Job drawing, mm, ordinate dimensions from the low corner. One solid piece. A direction names the side the tool comes from. Coordinates: 2 decimals unless noted, no trailing zeros. Order: outer loops, then holes, each group sorted by start corner. A loop starts at its lowest first (then second) coordinate and runs counter-clockwise, first axis right, second up. Notation, with made-up numbers: (47, 0.5) -> (78, 0.5) arc R21 cw to (78, 8.5) -> close; hole circle Ø10 at (58, 61). An arc over 180 degrees is marked (long way). Use CSV: the item, a comma, the result in double quotes. Start each with the question number.
(1) Cut at B-B on y = 2.85. Write the cut outline in (x, z) (1 decimal).
(2) Probe L1, parallel to Z at x = 4.2, y = 4.2; L2, parallel to Z at x = 2.9, y = 5.7; L3, parallel to Y at x = 2.35, z = 10.25 (1 decimal). List the from-to ranges inside material, lowest first.
(3) Pull direction Y, two halves, no side cores. Call the marked faces 1, 2 and 3: pulls with the +Y half, pulls with the -Y half, needs draft (parallel to the pull), parting line crosses it, or undercut.
(4) Cut at C-C on z = 1.5. Write the cut outline in (x, y).
(5) Pin check, flat tips, straight feed: pin 1 Ø1.8 at (x, y) = (2.5, 3.5) entering from +Z; pin 2 Ø3 at (x, z) = (5, 8.5) entering from +Y. Stop position of each tip, or through.
(6) Cut at D-D on x = 0.6. Write the cut outline in (y, z), plus the area to 3 significant figures.
(7) Tool access for the marked faces 4, 5 and 6: list every direction of +Z, -Z, +X, -X, +Y, -Y with a clear straight run to the whole face (end or side of a thin tool).
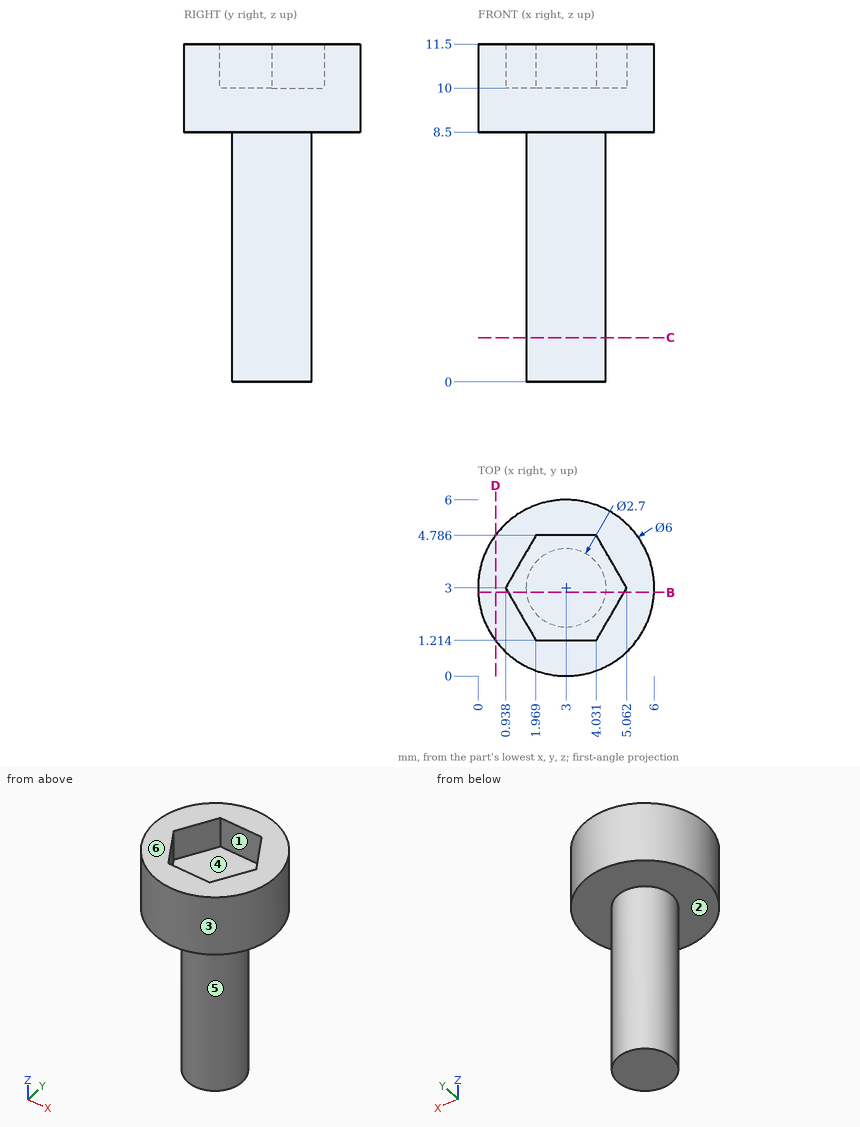
Outcome:
1,outline,"(0, 8.5) -> (1.7, 8.5) -> (1.7, 0) -> (4.3, 0) -> (4.3, 8.5) -> (6, 8.5) -> (6, 11.5) -> (5, 11.5) -> (5, 10) -> (1, 10) -> (1, 11.5) -> (0, 11.5) -> close"
2,L1,"8.5 to 10"
2,L2,"8.5 to 11.5"
2,L3,"0.1 to 1.2, 4.8 to 5.9"
3,face 1,"undercut"
3,face 2,"needs draft"
3,face 3,"parting line crosses it"
4,outline,"circle Ø2.7 at (3, 3)"
5,pin 1,"z = 10"
5,pin 2,"y = 5.96"
6,outline,"(1.2, 8.5) -> (4.8, 8.5) -> (4.8, 11.5) -> (1.2, 11.5) -> close"
6,area,"10.8 mm2"
7,face 4,"+Z"
7,face 5,"-Z"
7,face 6,"+Z, +X, -X, +Y, -Y"
